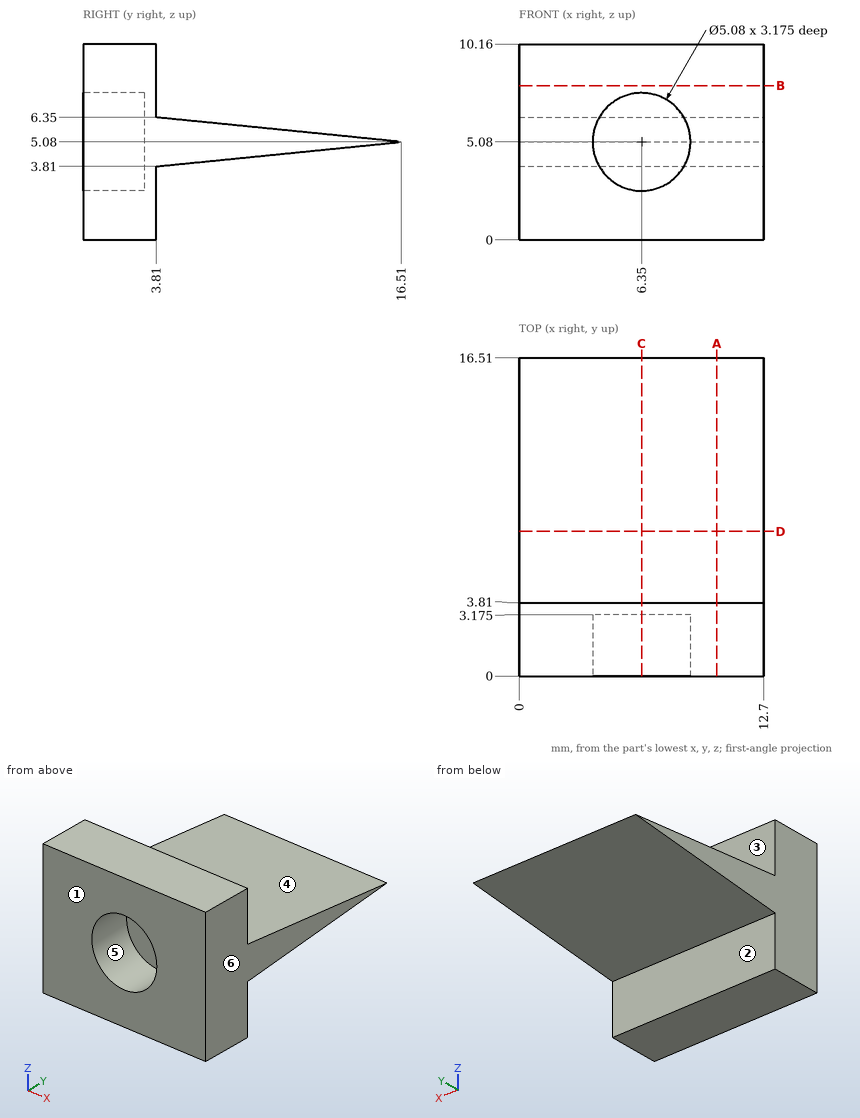
Geometry: see drawing. Coordinates: mm, zero at the bounding-box minimum. A direction names the side the tool comes from. Coordinates: 2 decimals unless noted, no trailing zeros. Loops run counter-clockwise (first coordinate to the right, second up) from the corner with the lowest first, then second, coordinate; pieces in that order, holes last. Notation, with made-up numbers: (84.5, 8) -> (127.5, 8) arc R32 ccw to (127.5, 37) -> close; hole circle Ø2 at (16, 71). An arc over 180 degrees is marked (long way). Use a Markdown table: item, result.
1) Material intervals for line 1 along Z through (x, y) = (6.35, 1.25); line 2 along Y through (x, z) = (7, 8); line 3 along Z through (x, y) = (2.25, 8.25), sorted ascending. Write a range as from..to.
Results found:
| item | result |
|---|---|
| line 1 | z = 0..2.54, 7.62..10.16 |
| line 2 | y = 0..3.81 |
| line 3 | z = 4.25..5.91 |
2) Cut plane D-D (y = 7.5). Return the cut outline in (x, z).
Results found:
| item | result |
|---|---|
| outline | (0, 4.18) -> (12.7, 4.18) -> (12.7, 5.98) -> (0, 5.98) -> close |
3) Contact query for flat-ended pins moving along their axis: pin 1 (1.5 mm diameter, centred on x = 5.5, z = 4.5, fed in from -Y) (3 decimals); pin 2 (5 mm diameter, centred on y = 11.5, z = 4, fed in from +X); pin 3 (3 mm diameter, centred on x = 2, z = 1.5, fed in from +Y). Output: stop coordinate, or through.
Results found:
| item | result |
|---|---|
| pin 1 | stops at y = 3.175 |
| pin 2 | stops at x = 12.7 |
| pin 3 | stops at y = 3.81 |
4) Access query for the marked faces 1, 2 and 3. Directions: +Z, -Z, +X, -X, +Y, -Y. A direction counts if a zero-diameter tool reaches every point of the face in a straight line with its end or side. Return the directions, or none.
Results found:
| item | result |
|---|---|
| face 1 | +Z, -Z, +X, -X, -Y |
| face 2 | -Z, +X, -X, +Y |
| face 3 | +Z, +X, -X, +Y |
5) Cut plane B-B (z = 8). Return the cut outline in (x, y).
Results found:
| item | result |
|---|---|
| outline | (0, 0) -> (12.7, 0) -> (12.7, 3.81) -> (0, 3.81) -> close |
6) Cut plane A-A (x = 10.25). Return the cut outline in (y, z), then the cut area to 3 significant figures.
Results found:
| item | result |
|---|---|
| outline | (0, 0) -> (3.81, 0) -> (3.81, 3.81) -> (16.51, 5.08) -> (3.81, 6.35) -> (3.81, 10.16) -> (0, 10.16) -> close |
| area | 54.8 mm2 |
7) Cut plane C-C (x = 6.35). Return the cut outline in (y, z) (3 decimals), then the cut area to 3 significant figures.
Results found:
| item | result |
|---|---|
| outline | (0, 0) -> (3.81, 0) -> (3.81, 3.81) -> (16.51, 5.08) -> (3.81, 6.35) -> (3.81, 10.16) -> (0, 10.16) -> (0, 7.62) -> (3.175, 7.62) -> (3.175, 2.54) -> (0, 2.54) -> close |
| area | 38.7 mm2 |
8) Pull-direction query (Z, two-part tool) for the marked faces 4, 5 and 6; classes: released by +Z, released by -Z, zero draft, split by the parting line, or undercut.
Results found:
| item | result |
|---|---|
| face 4 | released by +Z |
| face 5 | undercut |
| face 6 | zero draft |
